```python
from build123d import *

# Parameters (mm, degrees)
F1_DEPTH = 12


with BuildPart() as f1:
    # F0 (on Front) → F1 (new body)
    with BuildSketch(Plane.XZ):
        with BuildLine():
            Line((0, -9.5), (0, 7.5))
            Line((0, 7.5), (-9.5, 7.5))
            Line((-9.5, 7.5), (-9.5, 9.5))
            Line((-9.5, 9.5), (-13.5, 9.5))
            ThreePointArc((-13.5, 9.5), (-9.89512, 0.300815), (-1, -4))
            Line((-1, -4), (-1, -9.5))
            Line((-1, -9.5), (0, -9.5))
        make_face()
        Polygon((3, 9.5), (0, 9.5), (0, 7.5), (0, -9.5), (3, -9.5), align=None)
    extrude(amount=F1_DEPTH)


solid = f1.part
```
Can you work these out from the model? Positions are in its coordinate system, mm. A direction names the side the tool comes from. Coordinates: 2 decimals unless noted, no trailing zeros. Loops run counter-clockwise (first coordinate to the right, second up) from the corner with the lowest first, then second, coordinate; pieces in that order, holes last. Notation, with made-up numbers: (62.5, 79.25) - (118.5, 79.25) arc R13 cw to (118.5, 86.25) - close; hole circle Ø9 at (16.5, 31.25). An arc over 180 degrees is marked (long way). Use a Markdown table: item, result.
Item 1: If I drill on probe 1 along X at (y, z) = (-2, -8.5); probe 2 along Z at (x, y) = (-1.25, -9.5); probe 3 along Z at (x, y) = (-8.25, -3.5), over which ranges is the centre line in solid material (lowest first)? Write a range as from..to.
Numbers:
| item | result |
|---|---|
| probe 1 | x = -1..3 |
| probe 2 | z = -3.98..7.5 |
| probe 3 | z = -1.21..7.5 |
Item 2: I want a section at A-A on y = -4.25. Please give me the cut outline in (x, z), and give its area (3 significant figures).
Numbers:
| item | result |
|---|---|
| outline | (-13.5, 9.5) arc R13.54 ccw to (-1, -4) - (-1, -9.5) - (3, -9.5) - (3, 9.5) - (0, 9.5) - (0, 7.5) - (-9.5, 7.5) - (-9.5, 9.5) - close |
| area | 187 mm2 |
Item 3: I want a section at B-B on z = -7.75. Please give me the cut outline in (x, y).
Numbers:
| item | result |
|---|---|
| outline | (-1, -12) - (3, -12) - (3, 0) - (-1, 0) - close |
Item 4: For faces 1 (the face through (-4, 0, 2)), 2 (the face through (-5, -6, 7.5)), which set-ups out of +Z, -Z, +X, -X, +Y, -Y let a thin tool reach every point of the face, with its end or its side?
Numbers:
| item | result |
|---|---|
| face 1 | +Z, -Z, +X, -X, +Y |
| face 2 | +Z, +Y, -Y |
Item 5: Will these pins go through, and if not, where does the flat tip stop? pin 1 (2 mm diameter, centred on y = -6, z = 8.5, fed in from -X); pin 2 (4 mm diameter, centred on x = -6.5, y = -6.5, fed in from -Z); pin 3 (3 mm diameter, centred on x = -6, y = -6, fed in from +Z); pin 4 (5 mm diameter, centred on x = -6, y = -9, fed in from -Z).
Numbers:
| item | result |
|---|---|
| pin 1 | stops at x = -13.5 |
| pin 2 | stops at z = -3.26 |
| pin 3 | stops at z = 7.5 |
| pin 4 | stops at z = -3.57 |
Item 6: I want a section at C-C on x = -11. Please give me the cut outline in (y, z), and give its area (3 significant figures).
Numbers:
| item | result |
|---|---|
| outline | (-12, 1.66) - (0, 1.66) - (0, 9.5) - (-12, 9.5) - close |
| area | 94.1 mm2 |
Item 7: We'd pull the mould along X, two halves only. Please class faces 3 (the face through (2, -6, 9.5)), 4 (the face through (0, -6, 9)), 5 (the face through (-1, -6, -7)): released by +X, released by -X, zero draft, split by the parting line, or undercut.
Numbers:
| item | result |
|---|---|
| face 3 | zero draft |
| face 4 | undercut |
| face 5 | released by -X |
